```python
from build123d import *

# Parameters (mm, degrees)
CROQUIS1_R              = 2.25
SALIENTE_EXTRUIR1_DEPTH = 3


with BuildPart() as part:
    # Croquis1 → Saliente-Extruir1 (new body)
    with BuildSketch(Plane(origin=(0, 0, 0), x_dir=(-1, 0, 0), z_dir=(0, 0, 1))):
        with BuildLine():
            ThreePointArc((89.230623206, -116.44830451), (105.975312976, -80.770154924), (91.510495129, -44.10840322))
            add(Edge.make_bspline(
                [(91.510495129, -44.10840322), (84.127759627, -46.626480737), (76.659755812, -48.793582277), (61.567714608, -52.485529927), (53.943636753, -54.010209481), (42.395431338, -55.835856743), (38.534661436, -56.365996553), (30.807441475, -57.271160746), (26.938391186, -57.646594701), (15.315156999, -58.544821608), (7.544966548, -58.840628212), (-2.194410299, -58.832626174), (-4.144610508, -58.812018876), (-8.036264676, -58.733045352), (-9.978956608, -58.674697545), (-15.797685427, -58.443422776), (-19.664385347, -58.214324696), (-31.227228522, -57.302895154), (-38.886271373, -56.397367959), (-54.103241252, -53.978001601), (-61.66117651, -52.464211948), (-76.669501884, -48.789641951), (-84.119939601, -46.629147964), (-91.510495129, -44.10840322)],
                knots=[0, 0, 0, 0, 0.125, 0.125, 0.25, 0.25, 0.3125, 0.3125, 0.375, 0.375, 0.5, 0.5, 0.53125, 0.53125, 0.5625, 0.5625, 0.625, 0.625, 0.75, 0.75, 0.875, 0.875, 1, 1, 1, 1], degree=3))
            ThreePointArc((-91.510495129, -44.10840322), (-105.976396022, -80.735404374), (-89.282652322, -116.402173549))
            add(Edge.make_bspline(
                [(-89.282652322, -116.402173549), (-82.084427391, -118.871103079), (-74.801680613, -120.994537875), (-60.082232302, -124.612096128), (-52.645335382, -126.10542091), (-41.379555775, -127.893992917), (-37.614074487, -128.413191154), (-30.076442699, -129.300162486), (-26.302159817, -129.668099271), (-14.963168802, -130.548836526), (-7.382405934, -130.839774929), (2.120284858, -130.833963635), (4.022505287, -130.814238018), (7.817943392, -130.737887871), (13.501947355, -130.568056968), (19.158656691, -130.233305689), (30.435872975, -129.345060023), (37.90580458, -128.46158479), (52.74714565, -126.099341043), (60.118593514, -124.620804538), (74.756372315, -121.028591029), (82.022853845, -118.915823941), (89.230623206, -116.44830451)],
                knots=[0, 0, 0, 0, 0.125, 0.125, 0.25, 0.25, 0.3125, 0.3125, 0.375, 0.375, 0.5, 0.5, 0.53125, 0.53125, 0.5625, 0.625, 0.625, 0.75, 0.75, 0.875, 0.875, 1, 1, 1, 1], degree=3))
        make_face()
        with Locations(Location((90, -52.150876122, 0), (0, 0, 180))):
            Circle(CROQUIS1_R, mode=Mode.SUBTRACT)
        with Locations(Location((60, -118, 0), (0, 0, 180))):
            Circle(CROQUIS1_R, mode=Mode.SUBTRACT)
        with Locations(Location((-60, -118, 0), (0, 0, 180))):
            Circle(CROQUIS1_R, mode=Mode.SUBTRACT)
        with Locations(Location((-90, -52.150876122, 0), (0, 0, 180))):
            Circle(CROQUIS1_R, mode=Mode.SUBTRACT)
    extrude(amount=SALIENTE_EXTRUIR1_DEPTH)


solid = part.part
```
Geometry check sheet. Reference: the model listing, model coordinates, mm. Round coordinates to 2 decimals unless told otherwise and drop trailing zeros. Loops run counter-clockwise (first coordinate to the right, second up) from the corner with the lowest first, then second, coordinate; pieces in that order, holes last. Notation, with made-up numbers: (75.25, 85) - (105.25, 85) arc R12 ccw to (105.25, 105) - close; hole circle Ø11 at (-10, 76). An arc over 180 degrees is marked (long way). Write each question's results on one line, items separated by ' | '. Start each with the question number.
Q1. Cross-section at B-B on y = 113.5. Enter the section's corners in (x, z).
Q2. Gauge pin test, flat ends, axial feed: P1, Ø1.5, axis at y = 103, z = 2, coming from the -X side; P2, Ø4, axis at x = 90, y = 52.15, coming from the -Z side. Record the tip position at first contact, or that the pin passes through.
Q3. Thickness scan on line 1 (Y direction, x = -60, z = 1.5); line 2 (Y direction, x = -4.5, z = 0.5); line 3 (Y direction, x = 90, z = 0.7). Record the ranges inside material, lowest first. Write a range as [from, to].
Q4. Cross-section at A-A on z = 1.4. State how many separate pieces and enclosed holes the cut face has, and give its area (3 significant figures).
Q5. Cross-section at C-C on y = 95. Enter the section's corners in (x, z), and give its area (3 significant figures).
Answers below:
1) outline: (-92.29, 0) - (92.29, 0) - (92.29, 3) - (-92.29, 3) - close
2) P1: stops at x = -100.34 | P2: passes through
3) line 1: y = [52.71, 115.75], [120.25, 124.54] | line 2: y = [58.8, 130.8] | line 3: y = [44.62, 49.9], [54.4, 115.75]
4) separate pieces: 1 | enclosed holes: 4 | area: 14,500 mm²
5) outline: (-103.43, 0) - (103.43, 0) - (103.43, 3) - (-103.43, 3) - close | area: 621 mm²
